Here's how the part is built. I have some questions about the finished solid (model axes, mm). Face numbers are marked on the shaded views. A direction names the side the tool comes from. Give positions to 0.01 mm unless a question says otherwise; leave off trailing zeros. Loops run counter-clockwise (first coordinate to the right, second up) from the corner with the lowest first, then second, coordinate; pieces in that order, holes last. Notation, with made-up numbers: (9, 44.25) - (48, 44.25) arc R33 ccw to (48, 80.25) - close; hole circle Ø6 at (70, 68.25). An arc over 180 degrees is marked (long way). Use a Markdown table: item, result.
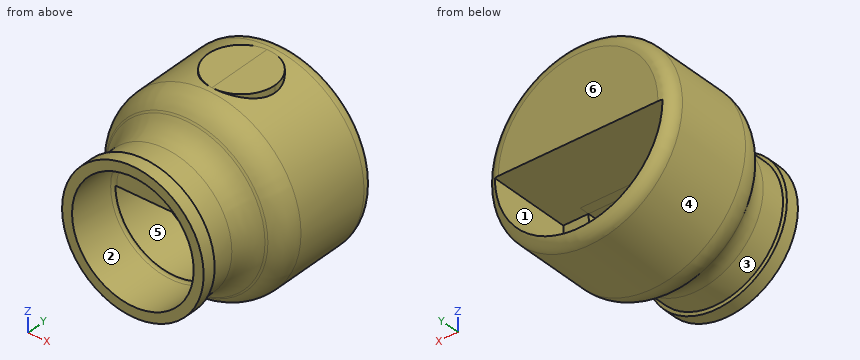
from build123d import *
from build123d.topology import SkipClean

# Parameters (mm, degrees)
CUT_EXTRUDE2_DEPTH      = 25
SKETCH10_R              = 10
BOSS_EXTRUDE1_DEPTH     = 5
CUT_EXTRUDE3_DEPTH      = 15
CUT_EXTRUDE3_DEPTH_BACK = 10


with BuildPart() as part:
    # Sketch1 → Revolve1 (revolve)
    with BuildSketch(Plane.XY):
        with BuildLine():
            Line((20.9, 0), (23.871591838, 0))
            Line((23.871591838, 0), (23.871591838, 4))
            Line((23.871591838, 4), (22.9, 4.236662843))
            Line((22.9, 4.236662843), (22.9, 11.404308102))
            ThreePointArc((22.9, 11.404308102), (23.83692213, 15.63049072), (26.472123903, 19.064752533))
            Line((26.472123903, 19.064752533), (26.988320528, 19.497892931))
            ThreePointArc((26.988320528, 19.497892931), (29.623522302, 22.932154745), (30.560444431, 27.158337362))
            Line((30.560444431, 27.158337362), (30.560444431, 50))
            ThreePointArc((30.560444431, 50), (29.388871556, 52.828427125), (26.560444431, 54))
            Line((26.560444431, 54), (2.764914955, 54))
            Line((2.764914955, 54), (2.764914955, 15))
            Line((2.764914955, 15), (19.9, 15))
            ThreePointArc((19.9, 15), (20.607106781, 14.707106781), (20.9, 14))
            Line((20.9, 14), (20.9, 0))
        make_face()
    revolve(axis=Axis((2.764914955, 7.821821657, 0), (0, 1, 0)))

    # Sketch9 → Cut-Extrude2 (cut)
    with BuildSketch(Plane(origin=(0, 54, 0), x_dir=(1, 0, 0), z_dir=(0, 1, 0))):
        with BuildLine():
            Line((-22.235085045, 0), (27.764914955, 0))
            ThreePointArc((27.764914955, 0), (2.764914955, 25), (-22.235085045, 0))
        make_face()
    extrude(amount=-CUT_EXTRUDE2_DEPTH, mode=Mode.SUBTRACT)

    # Sketch10 → Boss-Extrude1 (add)
    with SkipClean():  # the faces are left unmerged after this step: merging them gives an invalid solid
        with BuildSketch(Plane.XY.offset(27.795529476)):
            with Locations((3.346345887, 38.658337362)):
                Circle(SKETCH10_R)
        extrude(amount=-BOSS_EXTRUDE1_DEPTH)

    # Sketch11 → Cut-Extrude3 (cut, two sides: drawn at the far end of the back side and taken through both)
    with SkipClean():  # the faces are left unmerged after this step: merging them gives an invalid solid
        with BuildSketch(Plane(origin=(0, 17, 0), x_dir=(1, 0, 0), z_dir=(0, 1, 0)).offset(-CUT_EXTRUDE3_DEPTH_BACK)):
            with BuildLine():
                Line((-14.735085045, 0), (20.264914955, 0))
                ThreePointArc((20.264914955, 0), (2.764914955, 17.5), (-14.735085045, 0))
            make_face()
        extrude(amount=CUT_EXTRUDE3_DEPTH + CUT_EXTRUDE3_DEPTH_BACK, mode=Mode.SUBTRACT)


solid = part.part
(1) Suppose I cut it at A-A on y = 42.5. Write out the boundary of the cut face in (x, z).
A:
| item | result |
|---|---|
| outline | (-5.89, 26.41) arc R27.8 ccw (long way) to (12.58, 26.01) - (12.58, 27.8) - (-5.89, 27.8) - close; hole (-22.24, 0) arc R25 ccw to (27.76, 0) - close |
(2) If I drill on line 1 (Z direction, x = 3, y = 39); line 2 (X direction, y = 12, z = 0); line 3 (X direction, y = 31.5, z = -11), over which ranges is the centre line in solid material (lowest first)?
A:
| item | result |
|---|---|
| line 1 | -27.79 to -25, 0 to 27.8 |
| line 2 | -17.39 to -15.37, 20.9 to 22.92 |
| line 3 | -22.76 to -19.69, 25.21 to 28.29 |
(3) On a 3-axis mill with a long thin cutter (end or side, diameter ignored), from which of +Z, -Z, +X, -X, +Y, -Y can I reach the whole of each face in a straight line? I mean the marked faces 1, 2 and 3. Say none if no direction works.
A:
| item | result |
|---|---|
| face 1 | +Y |
| face 2 | -Y |
| face 3 | none |
(4) Suppose I cut it at B-B on y = 16. Write out the boundary of the cut face in (x, z).
A:
| item | result |
|---|---|
| outline | circle Ø42.51 at (2.76, 0); hole (-14.74, 0) arc R17.5 ccw to (20.26, 0) - close |
(5) We'd pull the mould along Z, two halves only. Please class the marked faces 4, 5 and 6: pulls with the +Z half, pulls with the -Z half, needs draft (parallel to the pull), parting line crosses it, or undercut.
A:
| item | result |
|---|---|
| face 4 | parting line crosses it |
| face 5 | undercut |
| face 6 | needs draft |
(6) Will these pins go through, and if not, where does the flat tip stop? pin 1 (12.5 mm diameter, centred on x = 7.5, y = 43, fed in from -Z); pin 2 (2 mm diameter, centred on y = 16.5, z = 4, fed in from -X); pin 3 (12 mm diameter, centred on y = 41, z = -9, fed in from +X).
A:
| item | result |
|---|---|
| pin 1 | z = -27.8 |
| pin 2 | x = -19.1 |
| pin 3 | x = 30.4 |
